Input: dimensioned drawing with shaded views. Units: mm. Origin: part minimum x, y, z. Coordinates: 2 decimals unless noted, no trailing zeros. Loops run counter-clockwise (first coordinate to the right, second up) from the corner with the lowest first, then second, coordinate; pieces in that order, holes last.
Item 1: Pin query (flat end, axial travel): pin 1 Ø6 at (x, y) = (112.5, 11.5) entering from -Z. Return the tip coordinate at first contact, or that it passes through.
Item 2: Section query D-D, the plane z = 72. Return the cut outline in (x, y), then the cut area to 3 significant figures.
Item 3: Line query: probe 1 along Z at (x, y) = (215.9, 3.25); probe 2 along X at (y, z) = (0.5, 37); probe 3 along X at (y, z) = (8.25, 54) (1 decimal). Output: solid intervals per line, ascending.
Item 4: Section query B-B, the plane z = 43.5. Return the cut outline in (x, y) (1 decimal), then the cut area to 3 significant figures.
Item 5: Section query C-C, the plane z = 13. Return the cut outline in (x, y), then the cut area to 3 significant figures.
Item 6: Section query A-A, the plane y = 9. Return the cut outline in (x, z), then the cut area to 3 significant figures.
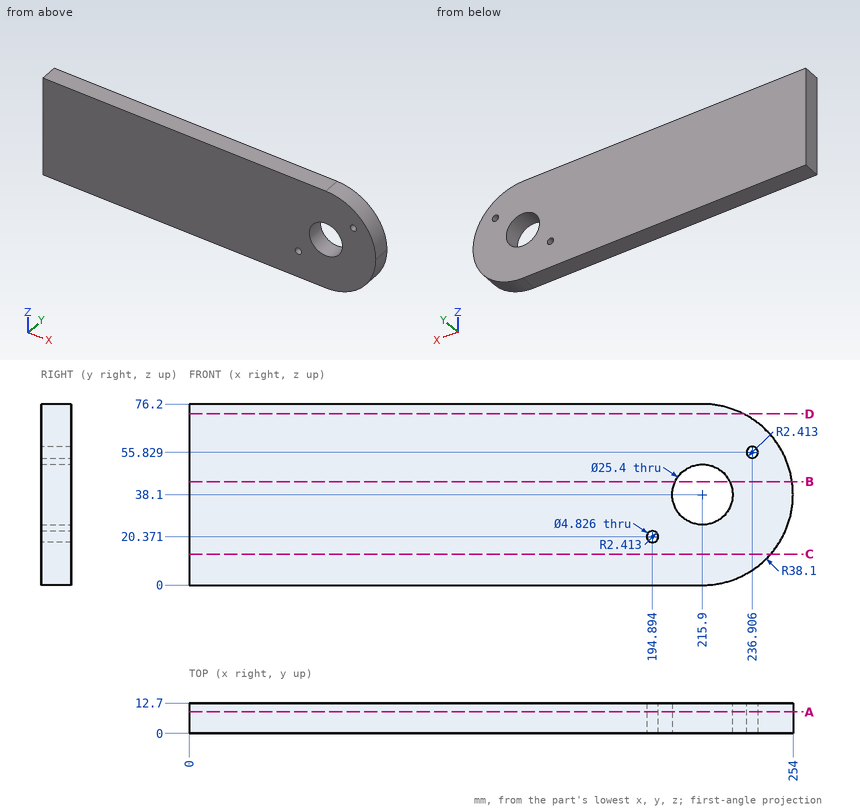
Verdict:
1. pin 1: stops at z = 0
2. outline: (0, 0) - (233.29, 0) - (233.29, 12.7) - (0, 12.7) - close
2. area: 2,960 mm2
3. probe 1: z = 0 to 25.4, 50.8 to 76.2
3. probe 2: x = 0 to 203.25, 228.55 to 253.98
3. probe 3: x = 0 to 235.3, 238.5 to 250.5
4. outline: (0, 0) - (204.4, 0) - (204.4, 12.7) - (0, 12.7) - close; (227.4, 0) - (253.6, 0) - (253.6, 12.7) - (227.4, 12.7) - close
4. area: 2,930 mm2
5. outline: (0, 0) - (244.56, 0) - (244.56, 12.7) - (0, 12.7) - close
5. area: 3,110 mm2
6. outline: (0, 0) - (215.9, 0) arc R38.1 ccw to (254, 38.1) arc R38.1 ccw to (215.9, 76.2) - (0, 76.2) - close; hole (194.89, 22.78) arc R2.41 ccw (long way) to (197.31, 20.37) arc R2.41 ccw to start; hole circle Ø25.4 at (215.9, 38.1); hole (234.49, 55.83) arc R2.41 ccw to (236.91, 53.42) arc R2.41 ccw to (239.32, 55.83) arc R2.41 ccw to start
6. area: 18,200 mm2
